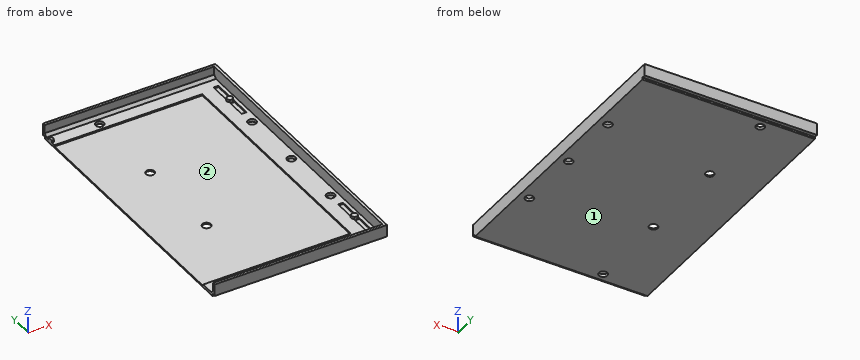
```python
from build123d import *

# Parameters (mm, degrees)
F0_W        = 245
F0_H        = 201
F1_DEPTH    = 8
F2_T        = -2
F3_W        = 210
F3_H        = 174
F4_DEPTH    = 1
F5_W        = 3.5
F5_H        = 33
F6_DEPTH    = 1
F8_W        = 3.5
F8_H        = 4.5
F9_DEPTH    = 1
F10_R       = 2.25
F11_DEPTH   = 1.5
F12_SIZE2   = 1.4896513151
F12_SIZE    = 0.15
F12_2_SIZE2 = 1.4896513151
F12_2_SIZE  = 0.15
F12_3_SIZE2 = 1.4896513151
F12_3_SIZE  = 0.15
F12_4_SIZE2 = 1.4896513151
F12_4_SIZE  = 0.15
F12_5_SIZE2 = 1.4896513151
F12_5_SIZE  = 0.15
F13_R       = 3
F14_DEPTH   = 2.001
F15_W       = 2.5
F15_H       = 1.5
F16_DEPTH   = 245.001
F17_SIZE    = 2
F18_DEPTH   = 2
F19_W       = 141.9361917675
F19_H       = 219.9546247721
F20_DEPTH   = 10.001


with BuildPart() as f1:
    # F0 (on Top) → F1 (new body)
    with BuildSketch(Plane.XY):
        with Locations((122.5, -100.5)):
            Rectangle(F0_W, F0_H)
    extrude(amount=F1_DEPTH)

    # F2
    f2_openings = [f1.faces().sort_by_distance(p)[0] for p in [
        (122.5, -100.5, 8),
    ]]
    offset(amount=F2_T, openings=f2_openings)

    # F3 (on face) → F4 (cut)
    with BuildSketch(Plane.XY.offset(2)):
        with Locations((122.5, -100.5)):
            Rectangle(F3_W, F3_H)
    extrude(amount=-F4_DEPTH, mode=Mode.SUBTRACT)

    # F5 (on face) → F6 (cut)
    with BuildSketch(Plane.XY.offset(2)):
        with Locations((6.25, -27.5)):
            Rectangle(F5_W, F5_H)
        with Locations((6.25, -173.5)):
            Rectangle(F5_W, F5_H)
        with Locations((238.75, -27.5)):
            Rectangle(F5_W, F5_H)
        with Locations((238.75, -173.5)):
            Rectangle(F5_W, F5_H)
    extrude(amount=-F6_DEPTH, mode=Mode.SUBTRACT)

    # F8 (on face) → F9 (join)
    with BuildSketch(Plane.XY.offset(2)):
        with Locations((238.75, -173.5)):
            Rectangle(F8_W, F8_H)
        with Locations((238.75, -27.5)):
            Rectangle(F8_W, F8_H)
        with Locations((6.25, -27.5)):
            Rectangle(F8_W, F8_H)
        with Locations((6.25, -173.5)):
            Rectangle(F8_W, F8_H)
    extrude(amount=-F9_DEPTH)

    # F10 (on face) → F11 (join)
    with BuildSketch(Plane.XY.offset(2)):
        with Locations((238.5, -27.5)):
            Circle(F10_R)
        with Locations((6.5, -27.5)):
            Circle(F10_R)
        with Locations((6.5, -173.5)):
            Circle(F10_R)
        with Locations((238.5, -173.5)):
            Circle(F10_R)
        with Locations((122.5, -8.5)):
            Circle(F10_R)
    extrude(amount=F11_DEPTH)

    # F12
    f12_edges = [f1.edges().sort_by_distance(p)[0] for p in [
        (236.25, -173.5, 3.5),
    ]]
    f12_side = f1.faces().sort_by_distance((238.5, -173.5, 3.5))[0]
    chamfer(f12_edges, length=F12_SIZE, length2=F12_SIZE2, reference=f12_side)

    # F12#2
    f12_2_edges = [f1.edges().sort_by_distance(p)[0] for p in [
        (4.25, -173.5, 3.5),
    ]]
    f12_2_side = f1.faces().sort_by_distance((6.5, -173.5, 3.5))[0]
    chamfer(f12_2_edges, length=F12_2_SIZE, length2=F12_2_SIZE2, reference=f12_2_side)

    # F12#3
    f12_3_edges = [f1.edges().sort_by_distance(p)[0] for p in [
        (236.25, -27.5, 3.5),
    ]]
    f12_3_side = f1.faces().sort_by_distance((238.5, -27.5, 3.5))[0]
    chamfer(f12_3_edges, length=F12_3_SIZE, length2=F12_3_SIZE2, reference=f12_3_side)

    # F12#4
    f12_4_edges = [f1.edges().sort_by_distance(p)[0] for p in [
        (4.25, -27.5, 3.5),
    ]]
    f12_4_side = f1.faces().sort_by_distance((6.5, -27.5, 3.5))[0]
    chamfer(f12_4_edges, length=F12_4_SIZE, length2=F12_4_SIZE2, reference=f12_4_side)

    # F12#5
    f12_5_edges = [f1.edges().sort_by_distance(p)[0] for p in [
        (120.25, -8.5, 3.5),
    ]]
    f12_5_side = f1.faces().sort_by_distance((122.5, -8.5, 3.5))[0]
    chamfer(f12_5_edges, length=F12_5_SIZE, length2=F12_5_SIZE2, reference=f12_5_side)

    # F13 (on face) → F14 (cut, through all)
    with BuildSketch(Plane.XY.offset(2)):
        with Locations((7, -54.5)):
            Circle(F13_R)
        with Locations((7, -100.5)):
            Circle(F13_R)
        with Locations((7, -146.5)):
            Circle(F13_R)
        with Locations((238, -54.5)):
            Circle(F13_R)
        with Locations((238, -100.5)):
            Circle(F13_R)
        with Locations((238, -146.5)):
            Circle(F13_R)
        with Locations((87.3, -8.5)):
            Circle(F13_R)
        with Locations((87.3, -67.5)):
            Circle(F13_R)
        with Locations((157.7, -8.5)):
            Circle(F13_R)
        with Locations((157.7, -67.5)):
            Circle(F13_R)
        with Locations((157.7, -133.5)):
            Circle(F13_R)
        with Locations((157.7, -192.5)):
            Circle(F13_R)
        with Locations((87.3, -192.5)):
            Circle(F13_R)
        with Locations((87.3, -133.5)):
            Circle(F13_R)
    extrude(amount=-F14_DEPTH, mode=Mode.SUBTRACT)

    # F15 (on face) → F16 (cut, through all)
    with BuildSketch(Plane(origin=(0, 0, 0), x_dir=(0, -1, 0), z_dir=(-1, 0, 0))):
        with Locations((1.25, 0.75)):
            Rectangle(F15_W, F15_H)
        with Locations((199.75, 0.75)):
            Rectangle(F15_W, F15_H)
    extrude(amount=-F16_DEPTH, mode=Mode.SUBTRACT)

    # F17
    f17_edges = [f1.edges().sort_by_distance(p)[0] for p in [
        (122.5, -2, 2),
        (122.5, -199, 2),
    ]]
    chamfer(f17_edges, length=F17_SIZE)

    # F18 (add): a face of the model
    f18_faces = [f1.faces().sort_by_distance(p)[0] for p in [
        (122.5, -0.3169006153, 8),
    ]]
    extrude(f18_faces, amount=F18_DEPTH)

    # F19 (on face) → F20 (cut, through all)
    with BuildSketch(Plane.XY.offset(10)):
        with Locations((51.5319041163, -105.3685471416)):
            Rectangle(F19_W, F19_H)
    extrude(amount=-F20_DEPTH, mode=Mode.SUBTRACT)


solid = f1.part
```
Model file for the job. Use its own axes, mm. Face numbers are marked on the shaded views. Coordinates: 2 decimals unless noted, no trailing zeros. Write each loop counter-clockwise with the first axis right and the second up, starting at its lowest first coordinate (ties: lowest second). Pieces come first, ordered by that corner, then holes. Notation, with made-up numbers: (50.25, -20.5) - (55.25, -20.5) arc R29 cw to (55.25, 9.5) - close; hole circle Ø9 at (-36.5, 63.25). An arc over 180 degrees is marked (long way). One line per item, written item: value. Start each with the question number.
1. Probe line 1 (Y direction, x = 238, z = 0.9); line 2 (X direction, y = -181.5, z = 1.5); line 3 (Y direction, x = 221.5, z = 7). List the from-to ranges inside material, lowest first. Write a range as from..to.
2. Slice it at C-C (y = -154). Write the cut outline in (x, z), plus the area to 3 significant figures.
3. Slice it at D-D (y = -67.5). Write the cut outline in (x, z), plus the area to 3 significant figures.
4. Mould opens along Y. For the marked faces 1 and 2 say: released by +Y, released by -Y, zero draft, split by the parting line, or undercut.
5. Slice it at A-A (y = -192.5). Write the cut outline in (x, z).
6. Slice it at B-B (x = 176). Write the cut outline in (y, z), plus the area to 4 significant figures.
7. Flat gauge pins, fed straight in: pin 1 (0.8 mm diameter, centred on y = -166, z = 1.5, fed in from -X); pin 2 (1.5 mm diameter, centred on x = 173.5, y = -127.5, fed in from +Z); pin 3 (9.5 mm diameter, centred on x = 157.7, y = -8.5, fed in from +Z). Where does each tip first touch, or does it go through?
Answers below:
1. line 1: y = -198.5..-149.5, -143.5..-103.5, -97.5..-57.5, -51.5..-2.5
1. line 2: x = 227.5..237, 240.5..245
1. line 3: y = -201..-199, -2..0
2. outline: (122.5, 0) - (245, 0) - (245, 10) - (243, 10) - (243, 2) - (227.5, 2) - (227.5, 1) - (122.5, 1) - close
2. area: 156 mm^2
3. outline: (122.5, 0) - (154.7, 0) - (154.7, 1) - (122.5, 1) - close; (160.7, 0) - (245, 0) - (245, 10) - (243, 10) - (243, 2) - (227.5, 2) - (227.5, 1) - (160.7, 1) - close
3. area: 150 mm^2
4. face 1: zero draft
4. face 2: undercut
5. outline: (122.5, 0) - (154.7, 0) - (154.7, 2) - (122.5, 2) - close; (160.7, 0) - (245, 0) - (245, 10) - (243, 10) - (243, 2) - (160.7, 2) - close
6. outline: (-201, 1.5) - (-198.5, 1.5) - (-198.5, 0) - (-2.5, 0) - (-2.5, 1.5) - (0, 1.5) - (0, 10) - (-2, 10) - (-2, 4) - (-4, 2) - (-13.5, 2) - (-13.5, 1) - (-187.5, 1) - (-187.5, 2) - (-197, 2) - (-199, 4) - (-199, 10) - (-201, 10) - close
6. area: 256.5 mm^2
7. pin 1: stops at x = 227.5
7. pin 2: stops at z = 1
7. pin 3: stops at z = 2.25
